```python
from build123d import *

# Parameters (mm, degrees)
F0_W      = 122.9868046939
F0_H      = 98.2980020344
F1_DEPTH  = 127
F2_W      = 80.4672054946
F2_H      = 81.8388015032
F3_DEPTH  = 127
F4_R      = 50.8
F5_R      = 20.2701316202
F6_DEPTH  = 254
F7_R      = 35.128731484
F8_DEPTH  = 25.4
F10_R     = 27.0682263701
F11_DEPTH = 25.4
F12_R     = 14.2572995328
F13_DEPTH = 50.8


with BuildPart() as f1:
    # F0 (on Right) → F1 (new body)
    with BuildSketch(Plane.YZ):
        with Locations((0.9144004434, 6.2865000218)):
            Rectangle(F0_W, F0_H)
    extrude(amount=F1_DEPTH)

    # F2 (on face) → F3 (cut)
    with BuildSketch(Plane.YZ.offset(127)):
        with Locations((1.6002003103, -1.9431002438)):
            Rectangle(F2_W, F2_H)
    extrude(amount=-F3_DEPTH, mode=Mode.SUBTRACT)

    # F4
    f4_edges = [f1.edges().sort_by_distance(p)[0] for p in [
        (127, -49.606202, -42.862501),
        (0, -49.606202, -42.862501),
        (0, 52.120803, -42.862501),
        (127, 52.120803, -42.862501),
    ]]
    fillet(f4_edges, radius=F4_R)

    # F5 (on face) → F6 (cut)
    with BuildSketch(Plane.XZ.offset(60.5790019035)):
        with Locations((62.1665008366, -9.2392507941)):
            Circle(F5_R)
    extrude(amount=-F6_DEPTH, mode=Mode.SUBTRACT)

    # F7 (on face) → F8 (join)
    with BuildSketch(Plane.XY.offset(55.435501039)):
        with Locations((63.5, 0)):
            Circle(F7_R)
    extrude(amount=F8_DEPTH)

    # F10 (on face) → F11 (cut)
    with BuildSketch(Plane.XY.offset(80.835501039)):
        with Locations((63.2483810186, 0)):
            Circle(F10_R)
    extrude(amount=-F11_DEPTH, mode=Mode.SUBTRACT)

    # F12 (on face) → F13 (cut)
    with BuildSketch(Plane.XY.offset(80.835501039)):
        with Locations((63.6905059218, 0)):
            Circle(F12_R)
    extrude(amount=-F13_DEPTH, mode=Mode.SUBTRACT)


solid = f1.part
```
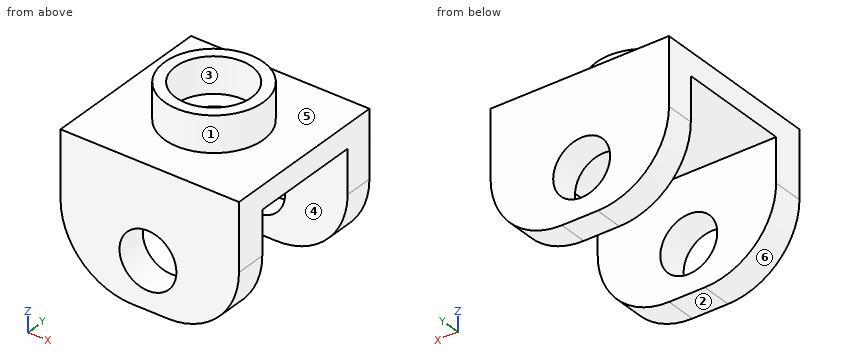
Source: CAD feature listing. Evaluate the final solid. Frame: model axes, mm. Face numbers are marked on the shaded views. A direction names the side the tool comes from. Give positions to 0.01 mm unless a question says otherwise; leave off trailing zeros. Loops run counter-clockwise (first coordinate to the right, second up) from the corner with the lowest first, then second, coordinate; pieces in that order, holes last. Notation, with made-up numbers: (67.5, 86) -> (105.5, 86) arc R22 cw to (105.5, 107) -> close; hole circle Ø3 at (-4.5, -28.5). An arc over 180 degrees is marked (long way). Put each result on its own line as item: value. Start each with the question number.
1) Cut plane B-B (z = 22). Return loops of the section in (x, y).
2) Cut plane A-A (y = 0). Return loops of the section in (x, z), then the cut area to 3 significant figures.
3) Contact query for flat-ended pins moving along their axis: P1, Ø10, axis at x = 97, y = -22.5, coming from the -Z side; P2, Ø8, axis at x = 19, y = 40, coming from the +Z side; P3, Ø6, axis at x = 42, y = -44, coming from the -Z side; P4, Ø17, axis at x = 63.69, y = 0, coming from the +Z side. Output: stop coordinate, or through.
4) Cut plane C-C (x = 63.5). Return loops of the section in (y, z).
5) Cut plane D-D (z = 2). Return loops of the section in (x, y).
6) Reachability of the marked faces 4, 5 and 6 from +Z, -Z, +X, -X, +Y, -Y: full face, straight path, thin tool, end or side. Return the list, or none.
7) Material intervals for probe 1 along Y at (x, z) = (77.5, 23); probe 2 along Z at (x, y) = (76.5, -9); probe 3 along X at (y, z) = (-6.5, 68.5), sorted ascending.
8) Draft query along Y for the marked faces 1, 2 and 3. Return one class per face: released by +Y, released by -Y, zero draft, split by the parting line, or undercut.
Results are:
1. outline: (0, -60.58) -> (127, -60.58) -> (127, -38.63) -> (0, -38.63) -> close; (0, 41.83) -> (127, 41.83) -> (127, 62.41) -> (0, 62.41) -> close
2. outline: (0, 38.98) -> (49.43, 38.98) -> (49.43, 55.44) -> (36.18, 55.44) -> (36.18, 80.84) -> (28.37, 80.84) -> (28.37, 55.44) -> (0, 55.44) -> close; (77.95, 38.98) -> (127, 38.98) -> (127, 55.44) -> (98.63, 55.44) -> (98.63, 80.84) -> (90.32, 80.84) -> (90.32, 55.44) -> (77.95, 55.44) -> close
2. area: 2,030 mm2
3. P1: stops at z = 38.98
3. P2: stops at z = 55.44
3. P3: stops at z = -42.53
3. P4: passes through
4. outline: (-60.58, -42.86) -> (-38.63, -42.86) -> (-38.63, -29.47) -> (-60.58, -29.47) -> close; (-60.58, 10.99) -> (-38.63, 10.99) -> (-38.63, 38.98) -> (-14.26, 38.98) -> (-14.26, 55.44) -> (-27.07, 55.44) -> (-27.07, 80.84) -> (-35.13, 80.84) -> (-35.13, 55.44) -> (-60.58, 55.44) -> close; (14.26, 38.98) -> (41.83, 38.98) -> (41.83, 10.99) -> (62.41, 10.99) -> (62.41, 55.44) -> (35.13, 55.44) -> (35.13, 80.84) -> (27.07, 80.84) -> (27.07, 55.44) -> (14.26, 55.44) -> close; (41.83, -42.86) -> (62.41, -42.86) -> (62.41, -29.47) -> (41.83, -29.47) -> close
5. outline: (0.35, -60.58) -> (45.3, -60.58) -> (45.3, -38.63) -> (0.35, -38.63) -> close; (0.35, 41.83) -> (45.3, 41.83) -> (45.3, 62.41) -> (0.35, 62.41) -> close; (79.04, -60.58) -> (126.65, -60.58) -> (126.65, -38.63) -> (79.04, -38.63) -> close; (79.04, 41.83) -> (126.65, 41.83) -> (126.65, 62.41) -> (79.04, 62.41) -> close
6. face 4: -Z, +X, -X
6. face 5: +Z
6. face 6: -Z, -X, +Y, -Y
7. probe 1: y = -60.58 to -38.63, 41.83 to 62.41
7. probe 2: z = 38.98 to 55.44
7. probe 3: x = 28.98 to 36.97, 89.52 to 98.02
8. face 1: split by the parting line
8. face 2: zero draft
8. face 3: undercut
